Verification items for the finished model (mm, model axes). Face numbers are marked on the shaded views. A direction names the side the tool comes from. Round coordinates to 2 decimals unless told otherwise and drop trailing zeros. Loops run counter-clockwise (first coordinate to the right, second up) from the corner with the lowest first, then second, coordinate; pieces in that order, holes last. Notation, with made-up numbers: (74.25, 50) -> (117.25, 50) arc R33 cw to (117.25, 83) -> close; hole circle Ø7 at (66.5, 46). An arc over 180 degrees is marked (long way). Write item = value, one per line.
```python
from build123d import *

# Parameters (mm, degrees)
BOSS_EXTRUDE1_DEPTH = 24
BOSS_EXTRUDE2_DEPTH = 36
SKETCH3_W           = 67
SKETCH3_H           = 25
CUT_EXTRUDE2_DEPTH  = 15


with BuildPart() as part:
    # Sketch1 → Boss-Extrude1 (new body)
    with BuildSketch(Plane.XY):
        Polygon((0, -27), (0, 27), (8, 29.911761874), (42, 17.5), (80, 17.5), (80, -17.5), (42, -17.5), (8, -29.911761874), align=None)
    extrude(amount=BOSS_EXTRUDE1_DEPTH)

    # Sketch2 → Boss-Extrude2 (add, symmetric)
    with BuildSketch(Plane(origin=(0, 0, 0), x_dir=(1, 0, 0), z_dir=(0, 1, 0))):
        Polygon((8, 0), (8, -6), (28, -3), (28, 0), align=None)
    extrude(amount=BOSS_EXTRUDE2_DEPTH, both=True)

    # Sketch3 → Cut-Extrude2 (cut)
    with BuildSketch(Plane.XY.offset(24)):
        with Locations((43.5, -1.797832718)):
            Rectangle(SKETCH3_W, SKETCH3_H)
    extrude(amount=-CUT_EXTRUDE2_DEPTH, mode=Mode.SUBTRACT)


solid = part.part
```
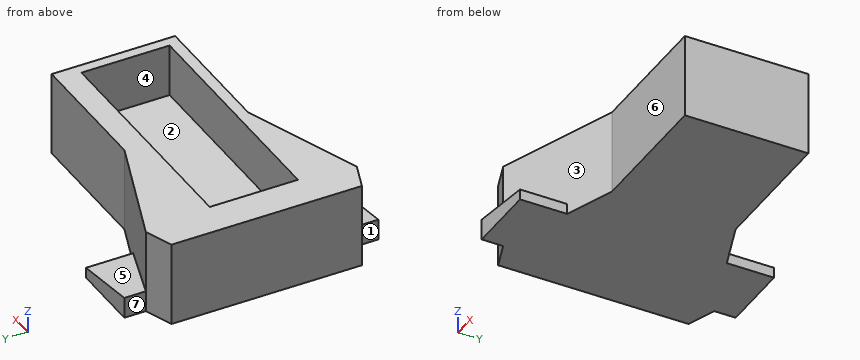
(1) Material ranges on probe 1 along X at (y, z) = (-3, 12.5); probe 2 along Y at (x, z) = (71.5, 16.25); probe 3 along Z at (x, y) = (34, -9), recorded low to high. Write a range as from..to.
Filled sheet:
probe_1 = 0..10, 77..80
probe_2 = -17.5..-14.3, 10.7..17.5
probe_3 = 0..9
(2) Sectioned sample at C-C, the plane y = -6. Record the cut outline in (x, z).
Filled sheet:
outline = (0, 0) -> (80, 0) -> (80, 24) -> (77, 24) -> (77, 9) -> (10, 9) -> (10, 24) -> (0, 24) -> close
(3) Sectioned sample at B-B, the plane x = 48. Record the cut outline in (y, z).
Filled sheet:
outline = (-17.5, 0) -> (17.5, 0) -> (17.5, 24) -> (10.7, 24) -> (10.7, 9) -> (-14.3, 9) -> (-14.3, 24) -> (-17.5, 24) -> close
(4) Set-up check for the marked faces 4, 5, 6 and 7: record each of +Z, -Z, +X, -X, +Y, -Y from which the full face is reachable in a straight line by a thin tool's end or side.
Filled sheet:
face_4 = +Z
face_5 = +Z, +X, +Y
face_6 = +Z, -Z, +X, -Y
face_7 = +Z, -Z, -X, +Y
(5) Sectioned sample at A-A, the plane z = 11.5. Record the cut outline in (x, y).
Filled sheet:
outline = (0, -27) -> (8, -29.91) -> (42, -17.5) -> (80, -17.5) -> (80, 17.5) -> (42, 17.5) -> (8, 29.91) -> (0, 27) -> close; hole (10, -14.3) -> (77, -14.3) -> (77, 10.7) -> (10, 10.7) -> close
(6) Draft check along X on the marked faces 1, 2 and 3. Enter one of: released by +X, released by -X, zero draft, split by the parting line, or undercut.
Filled sheet:
face_1 = released by -X
face_2 = undercut
face_3 = released by +X
(7) Go/stop test with flat-tipped pins: pin 1 Ø6 at (x, z) = (63.5, 18.5) entering from +Y; pin 2 Ø1.5 at (y, z) = (-31, 1.5) entering from +X; pin 3 Ø6.5 at (y, z) = (33.5, 3) entering from -X. Record where each tip stops, or that it passes through.
Filled sheet:
pin_1 = 17.5
pin_2 = 28
pin_3 = 8
(8) Sectioned sample at D-D, the plane z = 4.5. Record the cut outline in (x, y).
Filled sheet:
outline = (0, -27) -> (8, -29.91) -> (8, -36) -> (18, -36) -> (18, -26.26) -> (42, -17.5) -> (80, -17.5) -> (80, 17.5) -> (42, 17.5) -> (18, 26.26) -> (18, 36) -> (8, 36) -> (8, 29.91) -> (0, 27) -> close
